from build123d import *

# Parameters (mm, degrees)
PAD_DEPTH       = 40
SKETCH001_R     = 2.25
SKETCH001_R_2   = 4
POCKET_DEPTH    = 1.601
COPYSKETCH002_R = 2.25
POCKET001_DEPTH = 5


with BuildPart() as part:
    # Sketch → Pad (new body)
    with BuildSketch(Plane.XZ):
        Polygon((0, 0), (0, 40), (1.6, 40), (1.6, 1.6), (40, 1.6), (40, 0), align=None)
    extrude(amount=PAD_DEPTH)

    # Sketch001 (on Face3 of Pad) → Pocket (cut, through all)
    with BuildSketch(Plane(origin=(1.6, 0, 0), x_dir=(0, 0, 1), z_dir=(1, 0, 0))):
        with Locations((10.6, 35)):
            Circle(SKETCH001_R)
        with Locations((31, 25)):
            Circle(SKETCH001_R)
        with Locations((10.6, 15)):
            Circle(SKETCH001_R)
        with Locations((31, 5)):
            Circle(SKETCH001_R)
        with Locations((20, 20)):
            Circle(SKETCH001_R_2)
    extrude(amount=-POCKET_DEPTH, mode=Mode.SUBTRACT)

    # CopySketch002 → Pocket001 (cut)
    with BuildSketch(Plane(origin=(0, 0, 2.5), x_dir=(-1, 0, 0), z_dir=(0, 0, 1))):
        with Locations((-11.5, 5)):
            Circle(COPYSKETCH002_R)
        with Locations((-31, 15)):
            Circle(COPYSKETCH002_R)
        with Locations((-11.5, 25)):
            Circle(COPYSKETCH002_R)
        with Locations((-31, 35)):
            Circle(COPYSKETCH002_R)
    extrude(amount=-POCKET001_DEPTH, mode=Mode.SUBTRACT)


solid = part.part
Geometry: final body of the model. Coordinates: model frame, mm. A direction names the side the tool comes from. Give positions to 0.01 mm unless a question says otherwise; leave off trailing zeros. Write each loop counter-clockwise with the first axis right and the second up, starting at its lowest first coordinate (ties: lowest second). Pieces come first, ordered by that corner, then holes. Notation, with made-up numbers: (29, 23.5) - (58, 23.5) arc R9 cw to (58, 36.5) - close; hole circle Ø1 at (68, 16.5). An arc over 180 degrees is marked (long way). Return JSON: item names as keys, results as strings. Group by question number.
1) First-contact query: P1, Ø4, axis at y = -16, z = 17.5, coming from the +X side; P2, Ø10, axis at x = 32, z = 4.5, coming from the -Y side; P3, Ø2, axis at x = 28.5, y = -35.5, coming from the +Z side. Flat tips, straight axial feed; report the tip coordinate or a pass-through.
2) Section A-A on x = 11.5. Return the cut outline in (y, z), plus the area to 3 significant figures.
3) Section C-C on z = 21. Return the cut outline in (x, y).
4) Line query: line 1 (Y direction, x = 1, z = 31); line 2 (Z direction, x = 0.4, y = -25); line 3 (Y direction, x = 31, z = 1). Output: solid intervals per line, ascending.
5) Section B-B on y = -25. Return the cut outline in (x, z).
6) Mould query, pull axis Y, two halves, no side actions, for faces 1 (the cylindrical face through (0.811, -23.966, 19.479)), 2 (the flat face through (11, -40, 1)), 3 (the flat face through (11, 0, 1)), 4 (the flat face through (40, -20, 1)). Classes: released by +Y, released by -Y, zero draft, split by the parting line, or undercut.
7) Set-up query: faces 5 (the flat face through (0, -15, 20)), 6 (the flat face through (21, -20, 1.6)). Return all of +Z, -Z, +X, -X, +Y, -Y with unobstructed straight access to the full face (end or side cutting, diameter ignored); none if empty.
8) Section D-D on z = 31. Return the cut outline in (x, y), plus the area to 3 significant figures.
Filled in:
{
 "1": {"P1": "stops at x = 1.6", "P2": "stops at y = -40", "P3": "stops at z = 1.6"},
 "2": {"outline": "(-40, 0) - (-27.25, 0) - (-27.25, 1.6) - (-40, 1.6) - close; (-22.75, 0) - (-7.25, 0) - (-7.25, 1.6) - (-22.75, 1.6) - close; (-2.75, 0) - (0, 0) - (0, 1.6) - (-2.75, 1.6) - close", "area": "49.6 mm^2"},
 "3": {"outline": "(0, -40) - (1.6, -40) - (1.6, -23.87) - (0, -23.87) - close; (0, -16.13) - (1.6, -16.13) - (1.6, 0) - (0, 0) - close"},
 "4": {"line 1": "y = -40 to -27.25, -22.75 to -7.25, -2.75 to 0", "line 2": "z = 0 to 28.75, 33.25 to 40", "line 3": "y = -40 to -37.25, -32.75 to -17.25, -12.75 to 0"},
 "5": {"outline": "(0, 0) - (9.25, 0) - (9.25, 1.6) - (1.6, 1.6) - (1.6, 28.75) - (0, 28.75) - close; (0, 33.25) - (1.6, 33.25) - (1.6, 40) - (0, 40) - close; (13.75, 0) - (40, 0) - (40, 1.6) - (13.75, 1.6) - close"},
 "6": {"face 1": "undercut", "face 2": "released by -Y", "face 3": "released by +Y", "face 4": "zero draft"},
 "7": {"face 5": "+Z, -Z, -X, +Y, -Y", "face 6": "+Z, +X, +Y, -Y"},
 "8": {"outline": "(0, -40) - (1.6, -40) - (1.6, -27.25) - (0, -27.25) - close; (0, -22.75) - (1.6, -22.75) - (1.6, -7.25) - (0, -7.25) - close; (0, -2.75) - (1.6, -2.75) - (1.6, 0) - (0, 0) - close", "area": "49.6 mm^2"}
}
